Build history of the part. All positions in model axes, mm. A direction names the side the tool comes from. Round coordinates to 2 decimals unless told otherwise and drop trailing zeros. Order: outer loops, then holes, each group sorted by start corner. A loop starts at its lowest first (then second) coordinate and runs counter-clockwise, first axis right, second up. Notation, with made-up numbers: (65.25, 66.25) - (86.25, 66.25) arc R25 cw to (86.25, 84.25) - close; hole circle Ø1 at (-8.75, 71). An arc over 180 degrees is marked (long way). One line per question, with ' | ' between items. Start each with the question number.
from build123d import *

# Parameters (mm, degrees)
CROQUIS1_W              = 4.5
CROQUIS1_H              = 4.5
SALIENTE_EXTRUIR1_DEPTH = 2.5
CROQUIS2_R              = 1.75
CROQUIS2_R_2            = 1.1
CORTAR_EXTRUIR1_DEPTH   = 2.5


with BuildPart() as part:
    # Croquis1 → Saliente-Extruir1 (new body)
    with BuildSketch(Plane(origin=(0, 0, 0), x_dir=(1, 0, 0), z_dir=(0, 1, 0))):
        with BuildLine():
            ThreePointArc((-19.369757355, -2.25), (-13.788582233, -13.788582233), (-2.25, -19.369757355))
            Line((-2.25, -19.369757355), (-2.25, -15.335824073))
            ThreePointArc((-2.25, -15.335824073), (-10.960155108, -10.960155108), (-15.335824073, -2.25))
            Line((-15.335824073, -2.25), (-19.369757355, -2.25))
        make_face()
        with BuildLine():
            Line((-23.75, -2.25), (-19.369757355, -2.25))
            ThreePointArc((-19.369757355, -2.25), (-19.5, 0), (-19.369757355, 2.25))
            Line((-19.369757355, 2.25), (-23.75, 2.25))
            ThreePointArc((-23.75, 2.25), (-24.457106781, 1.957106781), (-24.75, 1.25))
            Line((-24.75, 1.25), (-24.75, -1.25))
            ThreePointArc((-24.75, -1.25), (-24.457106781, -1.957106781), (-23.75, -2.25))
        make_face()
        with BuildLine():
            Line((15.335824073, -2.25), (19.369757355, -2.25))
            ThreePointArc((19.369757355, -2.25), (19.467412109, -1.126883218), (19.5, 0))
            ThreePointArc((19.5, 0), (19.467412109, 1.126883218), (19.369757355, 2.25))
            Line((19.369757355, 2.25), (15.335824073, 2.25))
            ThreePointArc((15.335824073, 2.25), (15.458901532, 1.127990884), (15.5, 0))
            ThreePointArc((15.5, 0), (15.458901532, -1.127990884), (15.335824073, -2.25))
        make_face()
        with BuildLine():
            ThreePointArc((-19.369757355, 2.25), (-19.5, 0), (-19.369757355, -2.25))
            Line((-19.369757355, -2.25), (-15.335824073, -2.25))
            ThreePointArc((-15.335824073, -2.25), (-15.5, 0), (-15.335824073, 2.25))
            Line((-15.335824073, 2.25), (-19.369757355, 2.25))
        make_face()
        with BuildLine():
            Line((-2.25, 23.75), (-2.25, 19.369757355))
            ThreePointArc((-2.25, 19.369757355), (0, 19.5), (2.25, 19.369757355))
            Line((2.25, 19.369757355), (2.25, 23.75))
            ThreePointArc((2.25, 23.75), (1.957106781, 24.457106781), (1.25, 24.75))
            Line((1.25, 24.75), (-1.25, 24.75))
            ThreePointArc((-1.25, 24.75), (-1.957106781, 24.457106781), (-2.25, 23.75))
        make_face()
        with BuildLine():
            ThreePointArc((-2.25, 19.369757355), (-13.788582233, 13.788582233), (-19.369757355, 2.25))
            Line((-19.369757355, 2.25), (-15.335824073, 2.25))
            ThreePointArc((-15.335824073, 2.25), (-10.960155108, 10.960155108), (-2.25, 15.335824073))
            Line((-2.25, 15.335824073), (-2.25, 19.369757355))
        make_face()
        with BuildLine():
            ThreePointArc((-2.25, -19.369757355), (0, -19.5), (2.25, -19.369757355))
            Line((2.25, -19.369757355), (2.25, -15.335824073))
            ThreePointArc((2.25, -15.335824073), (0, -15.5), (-2.25, -15.335824073))
            Line((-2.25, -15.335824073), (-2.25, -19.369757355))
        make_face()
        with BuildLine():
            ThreePointArc((2.25, 19.369757355), (0, 19.5), (-2.25, 19.369757355))
            Line((-2.25, 19.369757355), (-2.25, 15.335824073))
            ThreePointArc((-2.25, 15.335824073), (0, 15.5), (2.25, 15.335824073))
            Line((2.25, 15.335824073), (2.25, 19.369757355))
        make_face()
        with BuildLine():
            Line((15.335824073, 2.25), (19.369757355, 2.25))
            ThreePointArc((19.369757355, 2.25), (13.788582233, 13.788582233), (2.25, 19.369757355))
            Line((2.25, 19.369757355), (2.25, 15.335824073))
            ThreePointArc((2.25, 15.335824073), (10.960155108, 10.960155108), (15.335824073, 2.25))
        make_face()
        with BuildLine():
            ThreePointArc((19.5, 0), (19.467412109, -1.126883218), (19.369757355, -2.25))
            Line((19.369757355, -2.25), (23.75, -2.25))
            ThreePointArc((23.75, -2.25), (24.457106781, -1.957106781), (24.75, -1.25))
            Line((24.75, -1.25), (24.75, 1.25))
            ThreePointArc((24.75, 1.25), (24.457106781, 1.957106781), (23.75, 2.25))
            Line((23.75, 2.25), (19.369757355, 2.25))
            ThreePointArc((19.369757355, 2.25), (19.467412109, 1.126883218), (19.5, 0))
        make_face()
        with BuildLine():
            Line((-1.25, -24.75), (1.25, -24.75))
            ThreePointArc((1.25, -24.75), (1.957106781, -24.457106781), (2.25, -23.75))
            Line((2.25, -23.75), (2.25, -19.369757355))
            ThreePointArc((2.25, -19.369757355), (0, -19.5), (-2.25, -19.369757355))
            Line((-2.25, -19.369757355), (-2.25, -23.75))
            ThreePointArc((-2.25, -23.75), (-1.957106781, -24.457106781), (-1.25, -24.75))
        make_face()
        with BuildLine():
            Line((2.25, -15.335824073), (2.25, -19.369757355))
            ThreePointArc((2.25, -19.369757355), (13.788582233, -13.788582233), (19.369757355, -2.25))
            Line((19.369757355, -2.25), (15.335824073, -2.25))
            ThreePointArc((15.335824073, -2.25), (10.960155108, -10.960155108), (2.25, -15.335824073))
        make_face()
        with BuildLine():
            ThreePointArc((-2.25, -15.335824073), (0, -15.5), (2.25, -15.335824073))
            Line((2.25, -15.335824073), (2.25, -2.25))
            Line((2.25, -2.25), (-2.25, -2.25))
            Line((-2.25, -2.25), (-2.25, -15.335824073))
        make_face()
        with BuildLine():
            Line((-15.335824073, -2.25), (-2.25, -2.25))
            Line((-2.25, -2.25), (-2.25, 2.25))
            Line((-2.25, 2.25), (-15.335824073, 2.25))
            ThreePointArc((-15.335824073, 2.25), (-15.5, 0), (-15.335824073, -2.25))
        make_face()
        with BuildLine():
            Line((-2.25, 2.25), (2.25, 2.25))
            Line((2.25, 2.25), (2.25, 15.335824073))
            ThreePointArc((2.25, 15.335824073), (0, 15.5), (-2.25, 15.335824073))
            Line((-2.25, 15.335824073), (-2.25, 2.25))
        make_face()
        Rectangle(CROQUIS1_W, CROQUIS1_H)
        with BuildLine():
            Line((2.25, 2.25), (2.25, -2.25))
            Line((2.25, -2.25), (15.335824073, -2.25))
            ThreePointArc((15.335824073, -2.25), (15.458901532, -1.127990884), (15.5, 0))
            ThreePointArc((15.5, 0), (15.458901532, 1.127990884), (15.335824073, 2.25))
            Line((15.335824073, 2.25), (2.25, 2.25))
        make_face()
    extrude(amount=SALIENTE_EXTRUIR1_DEPTH)

    # Croquis2 → Cortar-Extruir1 (cut)
    with BuildSketch(Plane(origin=(0, 2.5, 0), x_dir=(1, 0, 0), z_dir=(0, 1, 0))):
        with Locations(Location((0, 0, 0), (0, 0, 270))):
            Circle(CROQUIS2_R)
        with Locations(Location((-22.5, 0, 0), (0, 0, 270))):
            Circle(CROQUIS2_R_2)
        with Locations(Location((0, 22.5, 0), (0, 0, 270))):
            Circle(CROQUIS2_R_2)
        with Locations(Location((22.5, 0, 0), (0, 0, 270))):
            Circle(CROQUIS2_R_2)
        with Locations(Location((0, -22.5, 0), (0, 0, 270))):
            Circle(CROQUIS2_R_2)
    extrude(amount=-CORTAR_EXTRUIR1_DEPTH, mode=Mode.SUBTRACT)


solid = part.part
Item 1: Pull direction X, two halves, no side cores. Call faces 5 (the face through (2.25, 1, 22)), 6 (the face through (22, 1, -2.25)), 7 (the face through (9, 1, 2.25)): released by +X, released by -X, zero draft, split by the parting line, or undercut.
Item 2: Wall check: line 1 along X through (y, z) = (1.4, 0); line 2 along X through (y, z) = (0.3, 3); line 3 along Z through (x, y) = (3.5, 0.35). Give the ranges that are in metal, low to high. Write a range as [from, to].
Item 3: Slice it at A-A (z = 22.5). Write the cut outline in (x, y), plus the area to 3 significant figures.
Item 4: 3-axis set-ups, long thin cutter, end or side, ignore diameter. For faces 1 (the face through (22, 1, 2.25)), 2 (the face through (-2.25, 1, -22)), 3 (the face through (-22, 1, 2.25)), 4 (the face through (-9, 1, -2.25)): which of +Z, -Z, +X, -X, +Y, -Y reach the whole face in a straight line?
Item 5: Slice it at B-B (x = 0). Write the cut outline in (y, z).
Item 6: Slice it at D-D (z = 0). Write the cut outline in (x, y), plus the area to 3 significant figures.
Item 7: Slice it at C-C (x = -22.5). Write the cut outline in (y, z), plus the area to 3 significant figures.
Item 8: Pin check, flat tips, straight feed: pin 1 (1.2 mm diameter, centred on y = 1, z = -22.5, fed in from +X); pin 2 (1.2 mm diameter, centred on y = 1, z = 22, fed in from +X); pin 3 (1.2 mm diameter, centred on x = 22.5, y = 1.5, fed in from -Z). Stop position of each tip, or through.
A:
1) face 5: released by +X | face 6: zero draft | face 7: undercut
2) line 1: [-24.75, -23.6], [-21.4, -1.75], [1.75, 21.4], [23.6, 24.75] | line 2: [-19.27, -15.21], [-2.25, 2.25], [15.21, 19.27] | line 3: [-19.18, -15.1], [-2.25, 2.25], [15.1, 19.18]
3) outline: (-2.25, 0) - (-1.1, 0) - (-1.1, 2.5) - (-2.25, 2.5) - close; (1.1, 0) - (2.25, 0) - (2.25, 2.5) - (1.1, 2.5) - close | area: 5.75 mm^2
4) face 1: +Z, +X, +Y, -Y | face 2: -Z, -X, +Y, -Y | face 3: +Z, -X, +Y, -Y | face 4: +Y, -Y
5) outline: (0, -24.75) - (2.5, -24.75) - (2.5, -23.6) - (0, -23.6) - close; (0, -21.4) - (2.5, -21.4) - (2.5, -1.75) - (0, -1.75) - close; (0, 1.75) - (2.5, 1.75) - (2.5, 21.4) - (0, 21.4) - close; (0, 23.6) - (2.5, 23.6) - (2.5, 24.75) - (0, 24.75) - close
6) outline: (-24.75, 0) - (-23.6, 0) - (-23.6, 2.5) - (-24.75, 2.5) - close; (-21.4, 0) - (-1.75, 0) - (-1.75, 2.5) - (-21.4, 2.5) - close; (1.75, 0) - (21.4, 0) - (21.4, 2.5) - (1.75, 2.5) - close; (23.6, 0) - (24.75, 0) - (24.75, 2.5) - (23.6, 2.5) - close | area: 104 mm^2
7) outline: (0, -2.25) - (2.5, -2.25) - (2.5, -1.1) - (0, -1.1) - close; (0, 1.1) - (2.5, 1.1) - (2.5, 2.25) - (0, 2.25) - close | area: 5.75 mm^2
8) pin 1: x = 2.25 | pin 2: x = 2.25 | pin 3: z = -2.25
